Can you work these out from the model? Positions are in its coordinate system, mm. Give positions to 0.01 mm unless a question says otherwise; leave off trailing zeros. Order: outer loops, then holes, each group sorted by start corner. A loop starts at its lowest first (then second) coordinate and runs counter-clockwise, first axis right, second up. Notation, with made-up numbers: (86.5, 68.25) -> (94.5, 68.25) arc R32 cw to (94.5, 100.25) -> close; hole circle Ø2 at (39, 20.25). An arc over 180 degrees is marked (long way). Answer as a JSON object with one key per item and string values.
```python
from build123d import *

# Parameters (mm, degrees)
SKETCH1_R           = 0.5
BOSS_EXTRUDE1_DEPTH = 1


with BuildPart() as part:
    # Sketch1 → Boss-Extrude1 (new body)
    with BuildSketch(Plane.XY):
        with BuildLine():
            Line((1, 27), (2, 27))
            ThreePointArc((2, 27), (2.707106781, 26.707106781), (3, 26))
            Line((3, 26), (3, -26))
            ThreePointArc((3, -26), (2.707106781, -26.707106781), (2, -27))
            Line((2, -27), (1.5, -27))
            Line((1.5, -27), (1, -27))
            ThreePointArc((1, -27), (0.292893219, -26.707106781), (0, -26))
            Line((0, -26), (0, 26))
            ThreePointArc((0, 26), (0.292893219, 26.707106781), (1, 27))
        make_face()
        with Locations((1.5, 25.8)):
            Circle(SKETCH1_R, mode=Mode.SUBTRACT)
        with Locations((1.5, -25.8)):
            Circle(SKETCH1_R, mode=Mode.SUBTRACT)
    extrude(amount=BOSS_EXTRUDE1_DEPTH)


solid = part.part
```
1. If we section it at A-A on x = 1.5: Please give me the cut outline in (y, z), then the cut area to 3 significant figures.
Worked answers:
{"outline": "(-27, 0) -> (-26.3, 0) -> (-26.3, 1) -> (-27, 1) -> close; (-25.3, 0) -> (25.3, 0) -> (25.3, 1) -> (-25.3, 1) -> close; (26.3, 0) -> (27, 0) -> (27, 1) -> (26.3, 1) -> close", "area": "52.0 mm²"}
2. If we mould it in two halves opening along Y, with no side actions, what happens to faces 1 (the face through (2.699, 26.715, 0.493)), 2 (the face through (1.435, 26.296, 0.493)), 3 (the face through (2, 0, 0))? For each: +Y half, -Y half, draft (parallel to the pull), parting line (faces both ways), or undercut.
Worked answers:
{"face 1": "+Y half", "face 2": "undercut", "face 3": "draft"}
3. Please list where these lines run through material, in increasing order: L1, parallel to Y at x = 1.5, z = 0.7; L2, parallel to Y at x = 1.25, z = 0.3; L3, parallel to Y at x = 0.6, z = 0.3.
Worked answers:
{"L1": "-27 to -26.3, -25.3 to 25.3, 26.3 to 27", "L2": "-27 to -26.23, -25.37 to 25.37, 26.23 to 27", "L3": "-26.92 to 26.92"}
